For this review, take the finished solid that the model builds, in its own axes (mm). Give positions to 0.01 mm unless a question says otherwise; leave off trailing zeros. Order: outer loops, then holes, each group sorted by start corner. A loop starts at its lowest first (then second) coordinate and runs counter-clockwise, first axis right, second up. Notation, with made-up numbers: M 62,74 L 68,74 A18 cw 68,87 Z; hole C -38,-22 d11. An arc over 180 degrees is marked long. Answer as CSV lines item,"result". Start each with the question number.
1. For line 1 along Y through (x, z) = (0, 5.75); line 2 along Y through (x, z) = (-2, 1.75); line 3 along X through (y, z) = (-84.5, 1.75), list the stretches that pass through material, from the lowest coordinate up.
2. We need section D-D, the plane x = -89. Give the boundary of the cut face in (y, z).
3. Clearance check with flat-ended pins moving along their axes: P1, Ø21.5, axis at x = 90.91, y = 0, coming from the -Z side; P2, Ø1.5, axis at x = 43, z = 8, coming from the +Y side; P3, Ø1.5, axis at x = -33.5, z = 3, coming from the -Y side; P4, Ø2, axis at y = 38, z = 1.5, coming from the +X side. State where each tip first meets the part, or that it passes through.
4. We need section C-C, the plane y = 94.5. Give the boundary of the cut face in (x, z), and give its area (3 significant figures).
5. We need section A-A, the plane y = 0. Give the boundary of the cut face in (x, z), and give its area (3 significant figures).
6. We need section B-B, the plane x = 0. Give the boundary of the cut face in (y, z).
from build123d import *

# Parameters (mm, degrees)
SKETCH1_R               = 114.3
SKETCH1_R_2             = 49.149999464
EXTRUDE1_DEPTH          = 10.16
F_5_8_CLEARANCE_HOLE1_D = 16.66748


with BuildPart() as part:
    # Sketch1 → Extrude1 (new body)
    with BuildSketch(Plane.XY):
        Circle(SKETCH1_R)
        Circle(SKETCH1_R_2, mode=Mode.SUBTRACT)
    extrude(amount=EXTRUDE1_DEPTH)

    # 5/8 Clearance Hole1 (through all)
    with Locations(Plane(origin=(-61.229912904, -86.94526051, 0), x_dir=(-1, 0, 0), z_dir=(0, 0, -1))):
        with Locations((-61.229912904, 177.798020209), (29.681467244, 86.94526051), (-61.229912904, -3.966119638), (-152.141293051, 86.94526051)):
            Hole(F_5_8_CLEARANCE_HOLE1_D / 2)


solid = part.part
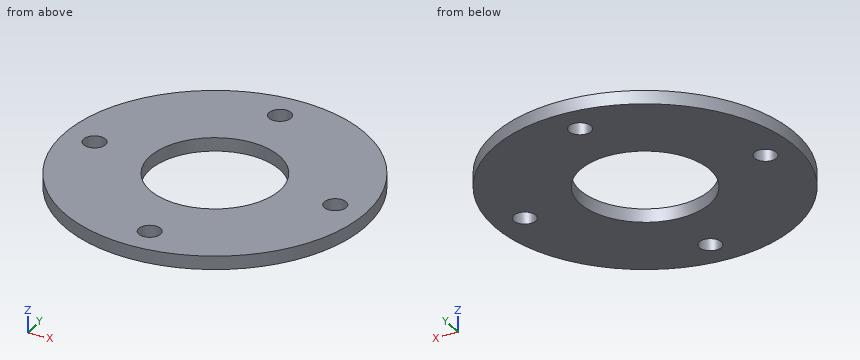
Result set:
1,line 1,"-114.3 to -99.25, -82.58 to -49.15, 49.15 to 82.52, 99.19 to 114.3"
1,line 2,"-114.28 to -99, -82.82 to -49.11, 49.11 to 82.76, 98.94 to 114.28"
1,line 3,"-76.97 to -5.32, 5.32 to 76.97"
2,outline,"M -71.72,0 L -8.11,0 L -8.11,10.16 L -71.72,10.16 Z; M 8.11,0 L 71.72,0 L 71.72,10.16 L 8.11,10.16 Z"
3,P1,"z = 0"
3,P2,"y = 106.2"
3,P3,"y = -109.51"
3,P4,"x = 108.15"
4,outline,"M -64.3,0 L -7.49,0 L -7.49,10.16 L -64.3,10.16 Z; M 7.49,0 L 64.3,0 L 64.3,10.16 L 7.49,10.16 Z"
4,area,"1,150 mm2"
5,outline,"M -114.3,0 L -99.25,0 L -99.25,10.16 L -114.3,10.16 Z; M -82.58,0 L -49.15,0 L -49.15,10.16 L -82.58,10.16 Z; M 49.15,0 L 82.58,0 L 82.58,10.16 L 49.15,10.16 Z; M 99.25,0 L 114.3,0 L 114.3,10.16 L 99.25,10.16 Z"
5,area,"985 mm2"
6,outline,"M -114.3,0 L -99.25,0 L -99.25,10.16 L -114.3,10.16 Z; M -82.58,0 L -49.15,0 L -49.15,10.16 L -82.58,10.16 Z; M 49.15,0 L 82.52,0 L 82.52,10.16 L 49.15,10.16 Z; M 99.19,0 L 114.3,0 L 114.3,10.16 L 99.19,10.16 Z"
